```python
from build123d import *

# Parameters (mm, degrees)
F1_DEPTH       = 7.9375
F3_D           = 12.7
F5_D           = 10.0838
F5_CSINK_D     = 19.8374
F5_CSINK_ANGLE = 82
F6_R           = 1.5875


with BuildPart() as f1:
    # F0 (on Top) → F1 (new body)
    with BuildSketch(Plane.XY):
        with BuildLine():
            Line((-46.0375, -46.0375), (23.5868596973, -46.0375))
            Line((23.5868596973, -46.0375), (47.5121798487, -69.9628201513))
            ThreePointArc((47.5121798487, -69.9628201513), (69.9628201513, -69.9628201513), (69.9628201513, -47.5121798487))
            Line((69.9628201513, -47.5121798487), (46.0375, -23.5868596973))
            Line((46.0375, -23.5868596973), (46.0375, 46.0375))
            Line((46.0375, 46.0375), (-46.0375, 46.0375))
            Line((-46.0375, 46.0375), (-46.0375, -46.0375))
        make_face()
    extrude(amount=F1_DEPTH)

    # F3 (through all)
    with Locations(Plane.XY.offset(7.9375)):
        with Locations((-33.3375, 33.3375), (-33.3375, -36.5125), (7.9375, -36.5125), (36.5125, -7.9375), (36.5125, 33.3375)):
            Hole(F3_D / 2)

    # F5 (through all)
    with Locations(Plane.XY.offset(7.9375)):
        with Locations((36.5125, -36.5125), (59.139916998, -59.139916998)):
            CounterSinkHole(F5_D / 2, F5_CSINK_D / 2, counter_sink_angle=F5_CSINK_ANGLE)

    # F6
    f6_edges = [f1.edges().sort_by_distance(p)[0] for p in [
        (-46.0375, -46.0375, 3.96875),
        (-46.0375, 46.0375, 3.96875),
        (46.0375, 46.0375, 3.96875),
        (46.0375, -23.58686, 3.96875),
        (23.58686, -46.0375, 3.96875),
    ]]
    fillet(f6_edges, radius=F6_R)


solid = f1.part
```
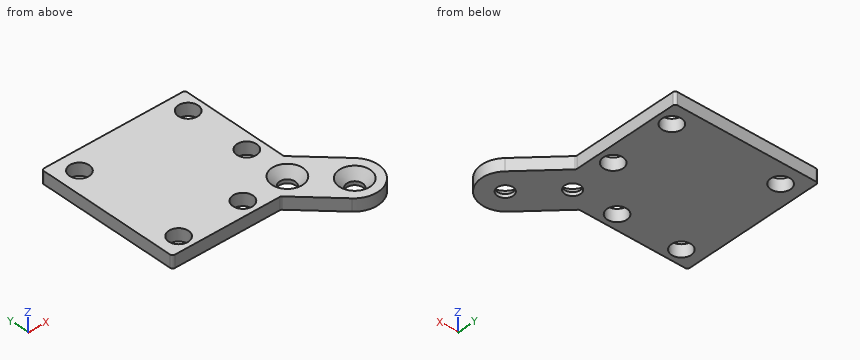
Model file for the job. Use its own axes, mm. Give positions to 0.01 mm unless a question says otherwise; leave off trailing zeros. Write each loop counter-clockwise with the first axis right and the second up, starting at its lowest first coordinate (ties: lowest second). Pieces come first, ordered by that corner, then holes. Notation, with made-up numbers: M -31.75,80 L -11.75,80 A19 cw -11.75,106 Z; hole C -14,-21.75 d4. An arc over 180 degrees is marked long. Use a Markdown table: item, result.
1) Cut at B-B (y = 9.5). List the corners of the cut face in (x, z), and give its area (3 significant figures).
Responses:
| item | result |
|---|---|
| outline | M -46.04,0 L 46.04,0 L 46.04,7.94 L -46.04,7.94 Z |
| area | 731 mm2 |
2) Cut at A-A (z = 4). Give the number of separate pieces and of enclosed holes in the cut face, and give its area (3 significant figures).
Responses:
| item | result |
|---|---|
| separate pieces | 1 |
| enclosed holes | 7 |
| area | 8,800 mm2 |
3) Pin check, flat tips, straight feed: pin 1 (8 mm diameter, centred on x = 59.14, y = -59.14, fed in from -Z); pin 2 (2 mm diameter, centred on y = -18, z = 6.5, fed in from +X). Stop position of each tip, or through.
Responses:
| item | result |
|---|---|
| pin 1 | passes through |
| pin 2 | stops at x = 46.04 |
4) Drill centre lines: line 1 (X direction, y = 31.5, z = 5.25); line 2 (X direction, y = -34, z = 6.75); line 3 (X direction, y = -37, z = 4.25). Where is each one in solid material? Low to high. Write a range as from..to.
Responses:
| item | result |
|---|---|
| line 1 | x = -46.04..-39.42, -27.26..30.43, 42.59..46.04 |
| line 2 | x = -46.04..-39.17, -27.51..2.11, 13.77..27.99, 45.04..56.45 |
| line 3 | x = -46.04..-39.67, -27.01..1.61, 14.27..29.82, 43.21..59.45 |
